from build123d import *

# Parameters (mm, degrees)
SKETCH1_R          = 7.5
EXTRUSION1_DEPTH   = 160
SKETCH2_R          = 2.25
EXTRUSION2_DEPTH   = 80
EXTRUSION3_START   = -10
EXTRUSION3_DEPTH   = 10
SKETCH4_R          = 9.988310786
EXTRUSION4_DEPTH   = 45
SKETCH5_R          = 7.5
SKETCH5_R_2        = 4
EXTRUSION5_DEPTH   = 15
SKETCH6_R          = 13.00139778
CUT_EXTRUDE1_DEPTH = 45


with BuildPart() as part:
    # Sketch1 → Extrusion1 (new body)
    with BuildSketch(Plane(origin=(0, 0, 0), x_dir=(-1, 0, 0), z_dir=(0, 1, 0))):
        with Locations(Location((0, 0, 0), (0, 0, 90))):
            Circle(SKETCH1_R)
    extrude(amount=EXTRUSION1_DEPTH)

    # Sketch2 → Extrusion2 (cut)
    with BuildSketch(Plane(origin=(0, 160, 0), x_dir=(-1, 0, 0), z_dir=(0, 1, 0))):
        with Locations(Location((0, 0, 0), (0, 0, 90))):
            Circle(SKETCH2_R)
    extrude(amount=-EXTRUSION2_DEPTH, mode=Mode.SUBTRACT)

    # Sketch3 → Extrusion3 (add)
    with BuildSketch(Plane(origin=(0, 160, 0), x_dir=(1, 0, 0), z_dir=(0, 1, 0)).offset(EXTRUSION3_START)):
        with BuildLine():
            Line((0, -7.5), (8, -7.5))
            Line((8, -7.5), (8, 7.5))
            Line((8, 7.5), (0, 7.5))
            ThreePointArc((0, 7.5), (7.5, 0), (0, -7.5))
        make_face()
    extrude(amount=EXTRUSION3_DEPTH)

    # Sketch4 → Extrusion4 (cut)
    with BuildSketch(Plane.XZ):
        Circle(SKETCH4_R)
    extrude(amount=-EXTRUSION4_DEPTH, mode=Mode.SUBTRACT)

    # Sketch5 → Extrusion5 (cut)
    with BuildSketch(Plane.XZ.offset(-45)):
        with Locations(Location((0, 0, 0), (0, 0, 270))):
            Circle(SKETCH5_R)
        with Locations(Location((0, 0, 0), (0, 0, 270))):
            Circle(SKETCH5_R_2, mode=Mode.SUBTRACT)
    extrude(amount=-EXTRUSION5_DEPTH, mode=Mode.SUBTRACT)

    # Sketch6 → Cut-Extrude1 (cut)
    with BuildSketch(Plane.XZ.offset(-45)):
        Circle(SKETCH6_R)
    extrude(amount=-CUT_EXTRUDE1_DEPTH, mode=Mode.SUBTRACT)


solid = part.part
Can you work these out from the model? Positions are in its coordinate system, mm. A direction names the side the tool comes from. Give positions to 0.01 mm unless a question says otherwise; leave off trailing zeros. Loops run counter-clockwise (first coordinate to the right, second up) from the corner with the lowest first, then second, coordinate; pieces in that order, holes last. Notation, with made-up numbers: (58.25, 47) - (69.25, 47) arc R24 cw to (69.25, 74) - close; hole circle Ø10 at (37.5, -31.5). An arc over 180 degrees is marked (long way). Return JSON: item names as keys, results as strings.
1. We'd pull the mould along Y, two halves only. Please class faces 4 (the face through (8, 155, 0)), 5 (the face through (2, 160, 2)), 6 (the face through (2, 90, 2)): +Y half, -Y half, draft (parallel to the pull), parting line (faces both ways), or undercut.
Output values:
{"face 4": "draft", "face 5": "+Y half", "face 6": "-Y half"}
2. I want a section at B-B on y = 139. Please give me the cut outline in (x, z), and give its area (3 significant figures).
Output values:
{"outline": "circle Ø15 at (0, 0); hole circle Ø4.5 at (0, 0)", "area": "161 mm²"}
3. I want a section at D-D on x = -6. Please give me the cut outline in (y, z), and give its area (3 significant figures).
Output values:
{"outline": "(90, -4.5) - (160, -4.5) - (160, 4.5) - (90, 4.5) - close", "area": "630 mm²"}
4. I'm going to push flat-ended pins straight in: pin 1 Ø1 at (x, y) = (2.5, 118.5) entering from -Z; pin 2 Ø1 at (x, y) = (5.5, 122.5) entering from -Z; pin 3 Ø3 at (x, y) = (-4.5, 150.5) entering from -Z. Where does each tip first touch, or does it pass through?
Output values:
{"pin 1": "stops at z = -7.23", "pin 2": "stops at z = -5.59", "pin 3": "stops at z = -6.87"}
5. I want a section at A-A on z = 0. Please give me the cut outline in (x, y), and give its area (3 significant figures).
Output values:
{"outline": "(-7.5, 90) - (-2.25, 90) - (-2.25, 160) - (-7.5, 160) - close; (2.25, 90) - (7.5, 90) - (7.5, 150) - (8, 150) - (8, 160) - (2.25, 160) - close", "area": "740 mm²"}
6. For faces 1 (the face through (-7.32, 124.51, -1.63)), 2 (the face through (0.676, 125.49, 2.146)), 3 (the face through (7.8, 150, -1.1)), which set-ups out of +Z, -Z, +X, -X, +Y, -Y let a thin tool reach every point of the face, with its end or its side?
Output values:
{"face 1": "-Y", "face 2": "+Y, -Y", "face 3": "+X, -Y"}
7. If I drill on line 1 (X direction, y = 119, z = 0); line 2 (X direction, y = 130.5, z = -2), over which ranges is the centre line in solid material (lowest first)?
Output values:
{"line 1": "x = -7.5 to -2.25, 2.25 to 7.5", "line 2": "x = -7.23 to -1.03, 1.03 to 7.23"}
